Design review of the part built by this model. Coordinates are the model's own, in mm. Coordinates: 2 decimals unless noted, no trailing zeros. Order: outer loops, then holes, each group sorted by start corner. A loop starts at its lowest first (then second) coordinate and runs counter-clockwise, first axis right, second up. Notation, with made-up numbers: M 70,-22.75 L 122,-22.75 A18 cw 122,-11.75 Z; hole C 46,48.5 d11. An arc over 180 degrees is marked long. Answer in a Markdown table with one row per item.
from build123d import *

# Parameters (mm, degrees)
F1_DEPTH = 6.35


with BuildPart() as f1:
    # F0 (on Front) → F1 (new body)
    with BuildSketch(Plane.XZ):
        with BuildLine():
            Line((-118.913364, 29.823589), (-115.967032, 29.823589))
            ThreePointArc((-115.967032, 29.823589), (-117.440198, 29.868968), (-118.913364, 29.823589))
        make_face()
        with BuildLine():
            Line((35.274541, 29.823589), (-115.967032, 29.823589))
            Line((-115.967032, 29.823589), (-118.913364, 29.823589))
            ThreePointArc((-118.913364, 29.823589), (-141.375006, 5.93416), (-118.913364, -17.955268))
            Line((-118.913364, -17.955268), (-115.967032, -17.955268))
            Line((-115.967032, -17.955268), (35.274541, -17.955268))
            Line((35.274541, -17.955268), (119.84679, -64.470268))
            Line((119.84679, -64.470268), (119.84679, 76.338588))
            Line((119.84679, 76.338588), (35.274541, 29.823589))
        make_face()
        with BuildLine():
            Line((-115.967032, -17.955268), (-118.913364, -17.955268))
            ThreePointArc((-118.913364, -17.955268), (-117.440198, -18.000648), (-115.967032, -17.955268))
        make_face()
    extrude(amount=F1_DEPTH)


solid = f1.part
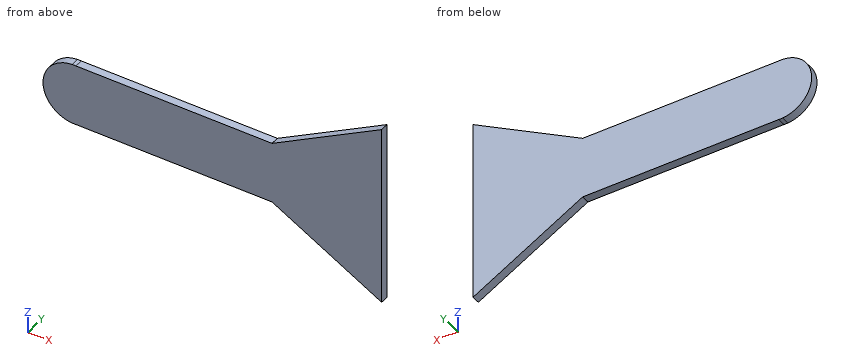
(1) Add section A-A, the plane y = -2.25. Give the boundary of the cut face in (x, z), and give its area (3 significant figures).
Return value:
| item | result |
|---|---|
| outline | M -118.91,-17.96 A23.93 ccw -115.97,-17.96 L 35.27,-17.96 L 119.85,-64.47 L 119.85,76.34 L 35.27,29.82 L -115.97,29.82 A23.93 ccw -118.91,29.82 A23.93 ccw Z |
| area | 16,200 mm2 |
(2) Add section C-C, the plane z = -48.5. Give the boundary of the cut face in (x, y).
Return value:
| item | result |
|---|---|
| outline | M 90.81,-6.35 L 119.85,-6.35 L 119.85,0 L 90.81,0 Z |
(3) Add section B-B, the plane x = 9. Give the boundary of the cut face in (y, z), and give its area (3 significant figures).
Return value:
| item | result |
|---|---|
| outline | M -6.35,-17.96 L 0,-17.96 L 0,29.82 L -6.35,29.82 Z |
| area | 303 mm2 |
(4) Insertion check: pin 1 Ø3 at (x, y) = (-8.5, -3.5) entering from -Z; pin 2 Ø3 at (x, y) = (82.5, -5.5) entering from -Z; pin 3 Ø2 at (x, y) = (-28, -5.5) entering from +Z. Each pin has a flat end and moves straight along its axis. Give the tip position at first contact, or say it passes through.
Return value:
| item | result |
|---|---|
| pin 1 | stops at z = -17.96 |
| pin 2 | stops at z = -44.75 |
| pin 3 | stops at z = 29.82 |
(5) For line 1 along Z through (x, y) = (-101.5, -1.75); line 2 along Z through (x, y) = (-127, -0.5); line 3 along X through (y, z) = (-1.75, 49), list the stretches that pass through material, from the lowest coordinate up. Write a range as from..to.
Return value:
| item | result |
|---|---|
| line 1 | z = -17.96..29.82 |
| line 2 | z = -16.01..27.88 |
| line 3 | x = 70.14..119.85 |
